Print and shaded views of the part. All mm, measured from the part's lowest x, y and z. A direction names the side the tool comes from. Give positions to 0.01 mm unless a question says otherwise; leave off trailing zeros. Loops run counter-clockwise (first coordinate to the right, second up) from the corner with the lowest first, then second, coordinate; pieces in that order, holes last. Notation, with made-up numbers: M -11.5,-23.75 L -4.5,-23.75 A35 ccw -4.5,12.25 Z; hole C 21,87.25 d10. An arc over 180 degrees is marked long. Answer as CSV lines item,"result".
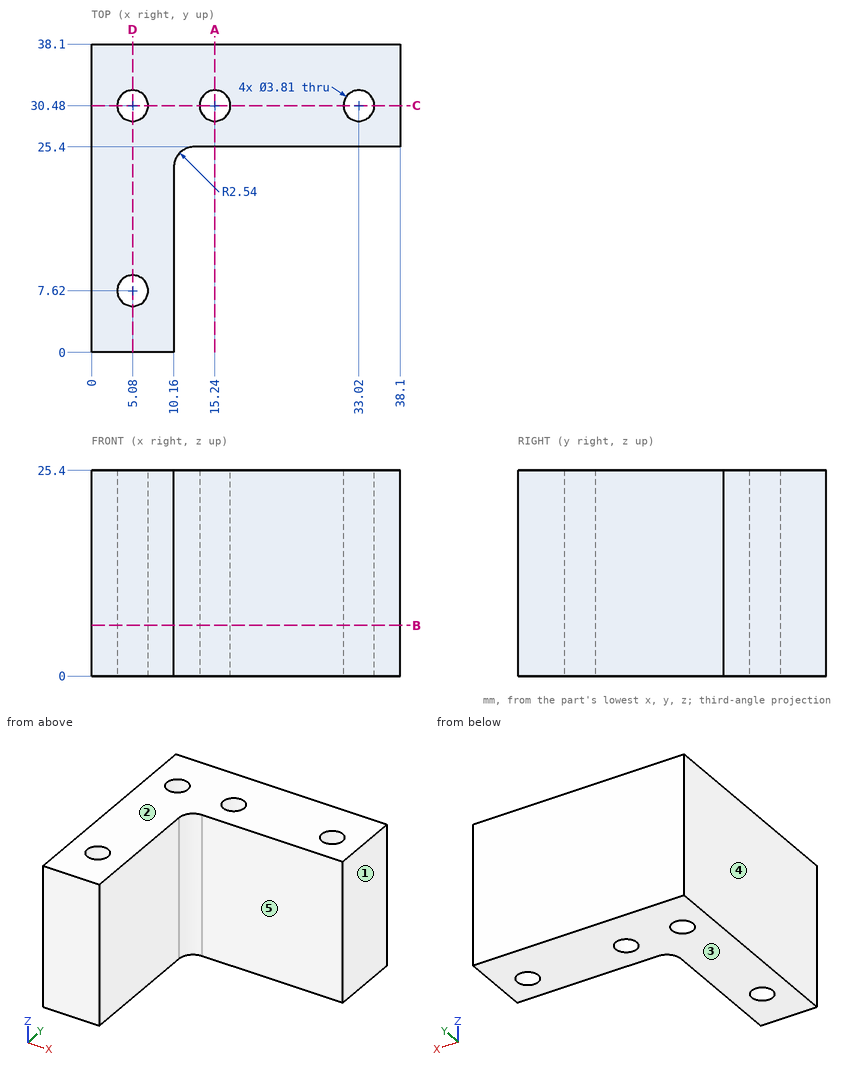
Q1. Cut at B-B (z = 6.25). Write the cut outline in (x, y) (3 decimals).
Solution:
outline,"M 0,0 L 10.16,0 L 10.16,22.86 A2.54 cw 12.7,25.4 L 38.1,25.4 L 38.1,38.1 L 0,38.1 Z; hole C 5.08,7.62 d3.81; hole C 5.08,30.48 d3.81; hole C 15.24,30.48 d3.81; hole C 33.02,30.48 d3.81"
Q2. Which spindle directions (+Z, -Z, +X, -X, +Y, -Y) get a long thin tool onto all of the face, cutting with end or side? Do the marked faces 4 and 5. Say none if no direction does.
Solution:
face 4,"+Z, -Z, -X, +Y, -Y"
face 5,"+Z, -Z, +X, -Y"
Q3. Cut at A-A (x = 15.24). Write the cut outline in (y, z) (3 decimals), and give its area (3 significant figures).
Solution:
outline,"M 25.4,0 L 28.575,0 L 28.575,25.4 L 25.4,25.4 Z; M 32.385,0 L 38.1,0 L 38.1,25.4 L 32.385,25.4 Z"
area,"226 mm²"
Q4. Mould opens along Z. For the marked faces 1, 2 and 3 say: released by +Z, released by -Z, zero draft, split by the parting line, or undercut.
Solution:
face 1,"zero draft"
face 2,"released by +Z"
face 3,"released by -Z"
Q5. Pin check, flat tips, straight feed: P1, Ø7.5, axis at x = 21.5, z = 11.5, coming from the -Y side; P2, Ø1.5, axis at y = 16.5, z = 14, coming from the +X side. Stop position of each tip, or through.
Solution:
P1,"stops at y = 25.4"
P2,"stops at x = 10.16"
Q6. Cut at C-C (y = 30.48). Write the cut outline in (x, z) (3 decimals).
Solution:
outline,"M 0,0 L 3.175,0 L 3.175,25.4 L 0,25.4 Z; M 6.985,0 L 13.335,0 L 13.335,25.4 L 6.985,25.4 Z; M 17.145,0 L 31.115,0 L 31.115,25.4 L 17.145,25.4 Z; M 34.925,0 L 38.1,0 L 38.1,25.4 L 34.925,25.4 Z"
Q7. Cut at D-D (x = 5.08). Write the cut outline in (y, z) (3 decimals), and give its area (3 significant figures).
Solution:
outline,"M 0,0 L 5.715,0 L 5.715,25.4 L 0,25.4 Z; M 9.525,0 L 28.575,0 L 28.575,25.4 L 9.525,25.4 Z; M 32.385,0 L 38.1,0 L 38.1,25.4 L 32.385,25.4 Z"
area,"774 mm²"
Q8. Wall check: line 1 (Y direction, x = 5.08, z = 15.25) (3 decimals); line 2 (Y direction, x = 4.5, z = 10.75); line 3 (X direction, y = 10, z = 14.25). Give the ranges that are in metal, low to high. Write a range as [from, to].
Solution:
line 1,"y = [0, 5.715], [9.525, 28.575], [32.385, 38.1]"
line 2,"y = [0, 5.81], [9.43, 28.67], [32.29, 38.1]"
line 3,"x = [0, 10.16]"
